Work out the finished part from the listing and answer in its coordinate system (mm). Face numbers are marked on the shaded views. A direction names the side the tool comes from. Coordinates: 2 decimals unless noted, no trailing zeros. Loops run counter-clockwise (first coordinate to the right, second up) from the corner with the lowest first, then second, coordinate; pieces in that order, holes last. Notation, with made-up numbers: (64.5, -14.5) - (91.5, -14.5) arc R10 cw to (91.5, -0.5) - close; hole circle Ø11 at (68.25, -31). An arc over 180 degrees is marked (long way). Write each question's results on one line, items separated by ' | '. Start each with the question number.
1. A cutting plane is placed at B-B on x = 12. Determine the outline of the cut face in (y, z).
2. Find the intervals of material crossed by line 1 along Y through (x, z) = (24, 1.55); line 2 along X through (y, z) = (0.75, 6); line 3 along Z through (x, y) = (-2.5, -1), in increasing order. Write a range as [from, to].
3. A cutting plane is placed at A-A on y = 1.5. Determine the outline of the cut face in (x, z).
4. Determine the mould class of the marked faces 4, 5, 6 and 7 for opening direction X: released by +X, released by -X, zero draft, split by the parting line, or undercut.
5. Each of these flat-tipped pins is pushed along its axis until it touches: P1, Ø2, axis at x = 8, y = 1.5, coming from the -Z side; P2, Ø4, axis at y = 0.5, z = 6, coming from the +X side; P3, Ø1.5, axis at y = 1, z = 7, coming from the +X side; P4, Ø2.5, axis at x = 2, y = 0.5, coming from the +Z side. Where does it stop, or does it pass through?
6. A cutting plane is placed at D-D on y = 3.25. Determine the outline of the cut face in (x, z), then the cut area to 3 significant figures.
7. Which of the six approach directions +Z, -Z, +X, -X, +Y, -Y give full straight-line access (tool end or side, diameter ignored) to the marked faces 1, 2 and 3?
8. A cutting plane is placed at C-C on z = 1. Determine the outline of the cut face in (x, y).
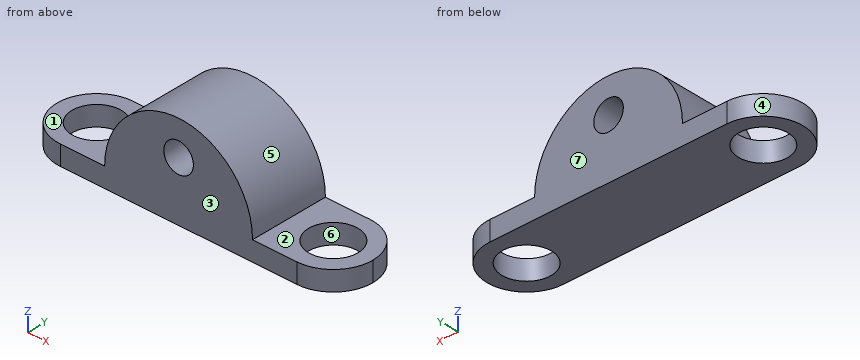
from build123d import *

# Parameters (mm, degrees)
BOSS_EXTRUDE1_DEPTH = 2
SKETCH2_R           = 1.5
BOSS_EXTRUDE2_DEPTH = 8
SKETCH6_R           = 2.5
CUT_EXTRUDE1_DEPTH  = 30.261749777


with BuildPart() as part:
    # Sketch1 → Boss-Extrude1 (new body)
    with BuildSketch(Plane.XY):
        with BuildLine():
            ThreePointArc((4, 0), (2.828427125, 2.828427125), (0, 4))
            Line((0, 4), (0, -4))
            ThreePointArc((0, -4), (2.828427125, -2.828427125), (4, 0))
        make_face()
        with BuildLine():
            Line((0, -4), (0, 4))
            ThreePointArc((0, 4), (-4, 0), (0, -4))
        make_face()
        with BuildLine():
            ThreePointArc((4, 0), (2.828427125, 2.828427125), (0, 4))
            Line((0, 4), (0, -4))
            ThreePointArc((0, -4), (2.828427125, -2.828427125), (4, 0))
        make_face()
        with BuildLine():
            Line((0, -4), (0, 4))
            ThreePointArc((0, 4), (-4, 0), (0, -4))
        make_face()
        with BuildLine():
            Line((24, 4), (0, 4))
            ThreePointArc((0, 4), (2.828427125, 2.828427125), (4, 0))
            ThreePointArc((4, 0), (2.828427125, -2.828427125), (0, -4))
            Line((0, -4), (24, -4))
            ThreePointArc((24, -4), (20, 0), (24, 4))
        make_face()
        with BuildLine():
            ThreePointArc((28, 0), (26.828427125, 2.828427125), (24, 4))
            Line((24, 4), (24, -4))
            ThreePointArc((24, -4), (26.828427125, -2.828427125), (28, 0))
        make_face()
        with BuildLine():
            Line((24, -4), (24, 4))
            ThreePointArc((24, 4), (20, 0), (24, -4))
        make_face()
        with BuildLine():
            ThreePointArc((28, 0), (26.828427125, 2.828427125), (24, 4))
            Line((24, 4), (24, -4))
            ThreePointArc((24, -4), (26.828427125, -2.828427125), (28, 0))
        make_face()
        with BuildLine():
            Line((24, -4), (24, 4))
            ThreePointArc((24, 4), (20, 0), (24, -4))
        make_face()
    extrude(amount=BOSS_EXTRUDE1_DEPTH)

    # Sketch2 → Boss-Extrude2 (add)
    with BuildSketch(Plane.XZ.offset(4)):
        with BuildLine():
            Line((4.5, 2), (19.5, 2))
            ThreePointArc((19.5, 2), (12, 9.5), (4.5, 2))
        make_face()
        with Locations(Location((12, 6, 0), (0, 0, 270))):
            Circle(SKETCH2_R, mode=Mode.SUBTRACT)
    extrude(amount=-BOSS_EXTRUDE2_DEPTH)

    # Sketch6 → Cut-Extrude1 (cut, through all)
    with BuildSketch(Plane.XY.offset(2)):
        Circle(SKETCH6_R)
        with Locations((24, 0)):
            Circle(SKETCH6_R)
    extrude(amount=-CUT_EXTRUDE1_DEPTH, mode=Mode.SUBTRACT)


solid = part.part
Values:
1) outline: (-4, 0) - (4, 0) - (4, 4.5) - (-4, 4.5) - close; (-4, 7.5) - (4, 7.5) - (4, 9.5) - (-4, 9.5) - close
2) line 1: [-4, -2.5], [2.5, 4] | line 2: [5.66, 10.5], [13.5, 18.34] | line 3: [0, 2]
3) outline: (-3.71, 0) - (-2, 0) - (-2, 2) - (-3.71, 2) - close; (2, 0) - (22, 0) - (22, 2) - (19.5, 2) arc R7.5 ccw to (4.5, 2) - (2, 2) - close; (26, 0) - (27.71, 0) - (27.71, 2) - (26, 2) - close; hole circle Ø3 at (12, 6)
4) face 4: released by -X | face 5: split by the parting line | face 6: undercut | face 7: zero draft
5) P1: z = 0 | P2: x = 19.23 | P3: x = 18.18 | P4: z = 2
6) outline: (-2.33, 0) - (26.33, 0) - (26.33, 2) - (19.5, 2) arc R7.5 ccw to (4.5, 2) - (-2.33, 2) - close; hole circle Ø3 at (12, 6) | area: 139 mm^2
7) face 1: +Z, -X, +Y, -Y | face 2: +Z, +X, +Y, -Y | face 3: +Z, -Z, +X, -X, -Y
8) outline: (0, -4) - (24, -4) arc R4 ccw to (24, 4) - (0, 4) arc R4 ccw to start; hole circle Ø5 at (0, 0); hole circle Ø5 at (24, 0)
